Check sheet for the modelled part. Datum: model origin and axes. Units: mm. Face numbers are marked on the shaded views. A direction names the side the tool comes from. Round coordinates to 2 decimals unless told otherwise and drop trailing zeros. Order: outer loops, then holes, each group sorted by start corner. A loop starts at its lowest first (then second) coordinate and runs counter-clockwise, first axis right, second up.
```python
from build123d import *

# Parameters (mm, degrees)
F0_R     = 7
F0_R_2   = 6
F1_DEPTH = 25
F3_START = 20
F3_DEPTH = 10


with BuildPart() as f1:
    # F0 (on Top) → F1 (new body)
    with BuildSketch(Plane.XY):
        with BuildLine():
            Line((-23.5798439344, -6.2340971038), (-10, 0))
            Line((-10, 0), (-23.5798439344, 6.2170174071))
            Line((-23.5798439344, 6.2170174071), (-59.8497580387, 3.4967738493))
            ThreePointArc((-59.8497580387, 3.4967738493), (-63.4999999675, -0.0004767763), (-59.8488053705, -3.496732787))
            Line((-59.8488053705, -3.496732787), (-23.5798439344, -6.2340971038))
        make_face()
        with BuildLine():
            ThreePointArc((-0.7525998222, -9.9716394594), (6.7997794735, -7.3323256277), (10, 0))
            ThreePointArc((10, 0), (7.0710678119, 7.0710678119), (0, 10))
            Line((0, 10), (-1.4916096955, 9.8881292728))
            ThreePointArc((-1.4916096955, 9.8881292728), (-4.2331341707, 9.059833061), (-6.6274556663, 7.4884465272))
            ThreePointArc((-6.6274556663, 7.4884465272), (-9.1179645937, 4.1064244384), (-10, 0))
            ThreePointArc((-10, 0), (-9.1094152791, -4.125354927), (-6.5962893453, -7.5159142407))
            ThreePointArc((-6.5962893453, -7.5159142407), (-3.8741695351, -9.2190460685), (-0.7525998222, -9.9716394594))
        make_face()
        Circle(F0_R, mode=Mode.SUBTRACT)
        Circle(F0_R)
        Circle(F0_R_2, mode=Mode.SUBTRACT)
        Circle(F0_R_2)
        with BuildLine():
            Line((-60, -5.5), (-0.7525998222, -9.9716394594))
            ThreePointArc((-0.7525998222, -9.9716394594), (-3.8741695351, -9.2190460685), (-6.5962893453, -7.5159142407))
            Line((-6.5962893453, -7.5159142407), (-23.5798439344, -6.2340971038))
            Line((-23.5798439344, -6.2340971038), (-59.8488053705, -3.496732787))
            Line((-59.8488053705, -3.496732787), (-60, -5.5))
        make_face()
        with BuildLine():
            ThreePointArc((-6.6274556663, 7.4884465272), (-4.2331341707, 9.059833061), (-1.4916096955, 9.8881292728))
            Line((-1.4916096955, 9.8881292728), (-60, 5.5))
            Line((-60, 5.5), (-59.8497580387, 3.4967738493))
            Line((-59.8497580387, 3.4967738493), (-23.5798439344, 6.2170174071))
            Line((-23.5798439344, 6.2170174071), (-6.6274556663, 7.4884465272))
        make_face()
        with BuildLine():
            Line((-23.5798439344, -6.2340971038), (-6.5962893453, -7.5159142407))
            ThreePointArc((-6.5962893453, -7.5159142407), (-9.1094152791, -4.125354927), (-10, 0))
            Line((-10, 0), (-23.5798439344, -6.2340971038))
        make_face()
        with BuildLine():
            ThreePointArc((-10, 0), (-9.1179645937, 4.1064244384), (-6.6274556663, 7.4884465272))
            Line((-6.6274556663, 7.4884465272), (-23.5798439344, 6.2170174071))
            Line((-23.5798439344, 6.2170174071), (-10, 0))
        make_face()
        with BuildLine():
            ThreePointArc((-60, 5.5), (-65.5, 0), (-60, -5.5))
            Line((-60, -5.5), (-59.8488053705, -3.496732787))
            ThreePointArc((-59.8488053705, -3.496732787), (-63.4999999675, -0.0004767763), (-59.8497580387, 3.4967738493))
            Line((-59.8497580387, 3.4967738493), (-60, 5.5))
        make_face()
        with BuildLine():
            Line((-1.4916096955, 9.8881292728), (0, 10))
            ThreePointArc((0, 10), (-0.7478994824, 9.9719930989), (-1.4916096955, 9.8881292728))
        make_face()
    extrude(amount=F1_DEPTH)

    # F2 (on Top) → F3 (cut)
    with BuildSketch(Plane.XY.offset(F3_START)):
        with BuildLine():
            ThreePointArc((-59, 3.5), (-56.5251262658, 2.4748737342), (-55.5, 0))
            ThreePointArc((-55.5, 0), (-56.5251262658, -2.4748737342), (-59, -3.5))
            Line((-59, -3.5), (-14.8914183851, -6.8290519661))
            Line((-14.8914183851, -6.8290519661), (-10, 0))
            Line((-10, 0), (-14.8914183851, 6.8081436211))
            Line((-14.8914183851, 6.8081436211), (-59, 3.5))
        make_face()
        with BuildLine():
            ThreePointArc((-59, -3.5), (-56.5251262658, -2.4748737342), (-55.5, 0))
            ThreePointArc((-55.5, 0), (-56.5251262658, 2.4748737342), (-59, 3.5))
            ThreePointArc((-59, 3.5), (-62.5, 0), (-59, -3.5))
        make_face()
    extrude(amount=F3_DEPTH, mode=Mode.SUBTRACT)


solid = f1.part
```
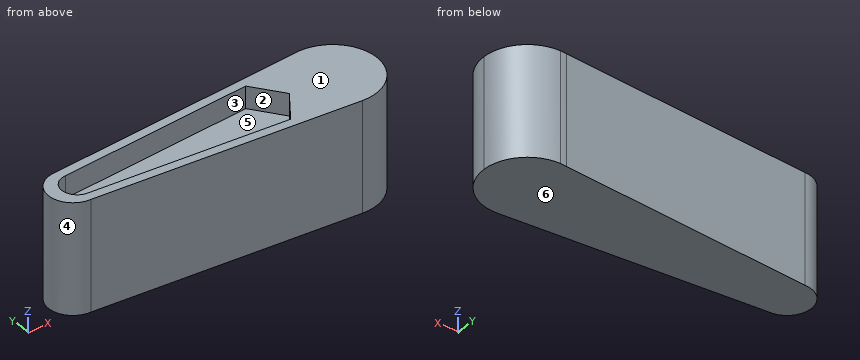
Item 1: Release check for a two-part mould opening along X. For the marked faces 3, 4, 5 and 6 record: released by +X, released by -X, zero draft, split by the parting line, or undercut.
Answer:
face 3: undercut
face 4: released by -X
face 5: undercut
face 6: zero draft
Item 2: Access from +Z, -Z, +X, -X, +Y, -Y to the whole of each face (thin tool, end or side, straight path). Record for the marked faces 1 and 2.
Answer:
face 1: +Z, +X, -X, +Y, -Y
face 2: +Z
Item 3: Sectioned sample at B-B (z = 23.25). Record the cut outline in (x, y), and give its area (3 significant figures).
Answer:
outline: (-60, -5.5) - (-0.75, -9.97) arc R10 ccw (long way) to (-1.49, 9.89) - (-60, 5.5) arc R5.5 ccw to start; hole (-59, -3.5) - (-14.89, -6.83) - (-10, 0) - (-14.89, 6.81) - (-59, 3.5) arc R3.5 ccw to start
area: 628 mm2
Item 4: Scan lines: line 1 along Z through (x, y) = (-16.5, 3); line 2 along X through (y, z) = (0.25, 4); line 3 along Y through (x, z) = (-60.5, 4.75). Record each from-to range of solid material in increasing order.
Answer:
line 1: z = 0 to 20
line 2: x = -65.49 to 10
line 3: y = -5.48 to 5.48
Item 5: Sectioned sample at C-C (y = -2). Record the cut outline in (x, z).
Answer:
outline: (-65.12, 0) - (9.8, 0) - (9.8, 25) - (-11.43, 25) - (-11.43, 20) - (-61.87, 20) - (-61.87, 25) - (-65.12, 25) - close
Item 6: Go/stop test with flat-tipped pins: P1, Ø10, axis at x = -12, z = 3.5, coming from the -Y side; P2, Ø7, axis at x = -29.5, y = 1.5, coming from the +Z side; P3, Ø1.5, axis at x = -15.5, z = 18, coming from the -Y side. Record where each tip stops, or that it passes through.
Answer:
P1: stops at y = -9.5
P2: stops at z = 20
P3: stops at y = -8.92
Item 7: Sectioned sample at A-A (z = 14.25). Record the cut outline in (x, y).
Answer:
outline: (-60, -5.5) - (-0.75, -9.97) arc R10 ccw (long way) to (-1.49, 9.89) - (-60, 5.5) arc R5.5 ccw to start
